```python
from build123d import *

# Parameters (mm, degrees)
F0_R     = 3.9497
F1_DEPTH = 6.0452
F0_R_2   = 11.4554
F2_DEPTH = 2.54
F3_R     = 1.016
F4_R     = 1.27
F5_R     = 4.2926
F5_R_2   = 3.9497
F6_DEPTH = 0.635


with BuildPart() as f1:
    # F0 (on Top) → F1 (new body)
    with BuildSketch(Plane.XY):
        Circle(F0_R)
    extrude(amount=F1_DEPTH)

    # F0 (on Top) → F2 (join)
    with BuildSketch(Plane.XY):
        Circle(F0_R_2)
        Circle(F0_R, mode=Mode.SUBTRACT)
    extrude(amount=F2_DEPTH)

    # F3
    f3_edges = [f1.edges().sort_by_distance(p)[0] for p in [
        (-11.4554, 0, 0),
    ]]
    fillet(f3_edges, radius=F3_R)

    # F4
    f4_edges = [f1.edges().sort_by_distance(p)[0] for p in [
        (-3.9497, 0, 6.0452),
    ]]
    fillet(f4_edges, radius=F4_R)

    # F5 (on face) → F6 (join)
    with BuildSketch(Plane.XY.offset(2.54)):
        Circle(F5_R)
        Circle(F5_R_2, mode=Mode.SUBTRACT)
    extrude(amount=F6_DEPTH)


solid = f1.part
```
Work out the finished part from the listing and answer in its coordinate system (mm). A direction names the side the tool comes from. Coordinates: 2 decimals unless noted, no trailing zeros. Order: outer loops, then holes, each group sorted by start corner. A loop starts at its lowest first (then second) coordinate and runs counter-clockwise, first axis right, second up. Notation, with made-up numbers: (33.5, -20.5) - (80.5, -20.5) arc R10 ccw to (80.5, -16.5) - close; hole circle Ø8 at (32, 80). An arc over 180 degrees is marked (long way). Answer as a JSON object with one key per item and string values.
1. Find section A-A on y = 0. Determine the outline of the cut face in (x, z) (3 decimals), plus the area to 3 significant figures.
Output values:
{"outline": "(-11.455, 1.016) arc R1.016 ccw to (-10.439, 0) - (10.439, 0) arc R1.016 ccw to (11.455, 1.016) - (11.455, 2.54) - (4.293, 2.54) - (4.293, 3.175) - (3.95, 3.175) - (3.95, 4.775) arc R1.27 ccw to (2.68, 6.045) - (-2.68, 6.045) arc R1.27 ccw to (-3.95, 4.775) - (-3.95, 3.175) - (-4.293, 3.175) - (-4.293, 2.54) - (-11.455, 2.54) - close", "area": "85.2 mm²"}
2. Consider line 1 (Z direction, x = -10, y = -0.5); line 2 (X direction, y = -3.5, z = 3.5); line 3 (Y direction, x = -6.5, z = 1.25). Determine where each line is inside the solid, lowest interval first.
Output values:
{"line 1": "z = 0 to 2.54", "line 2": "x = -1.83 to 1.83", "line 3": "y = -9.43 to 9.43"}
3. Find section C-C on z = 5.75. Determine the outline of the cut face in (x, y).
Output values:
{"outline": "circle Ø6.99 at (0, 0)"}
4. Each of these flat-tipped pins is pushed along its axis until it touches: P1, Ø1, axis at x = -5, z = 1, coming from the -Y side; P2, Ø7, axis at x = -3, y = -5.5, coming from the +Z side; P3, Ø4, axis at x = -6.5, y = 2.5, coming from the +Z side. Where does it stop, or does it pass through?
Output values:
{"P1": "stops at y = -10.53", "P2": "stops at z = 6.04", "P3": "stops at z = 2.54"}
5. A tool of negligible diameter and unlimited length cuts with its end or side. For faces 1 (the face through (-8.443, 7.742, 1.767)), 2 (the face through (4.094, 1.289, 2.853)), from which of +Z, -Z, +X, -X, +Y, -Y can it reach the whole face along a straight path? Write none if from no direction.
Output values:
{"face 1": "+Z, -Z", "face 2": "+Z"}
